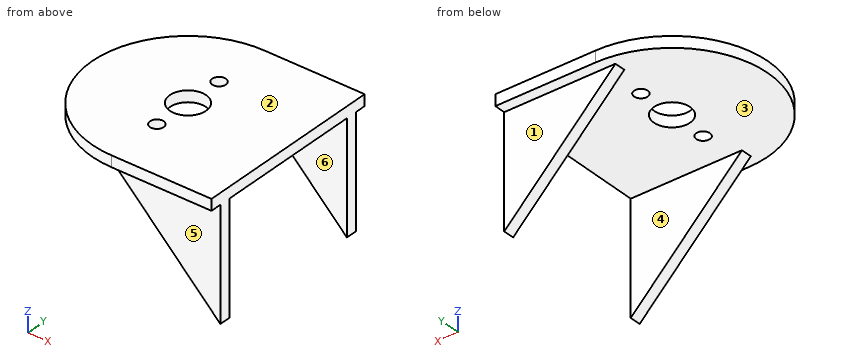
Autodesk Inventor part; units mm, degrees
ref_plane "YZ Plane" through (0, 0, 0) normal (1, 0, 0) x (0, 1, 0)
ref_plane "XZ Plane" through (0, 0, 0) normal (0, 1, 0) x (-1, 0, 0)
ref_plane "XY Plane" through (0, 0, 0) normal (0, 0, 1) x (1, 0, 0)
ref_plane "Płaszczyzna konstrukcyjna1" through (0, 0, 0) normal (0, 0, 1) x (1, 0, 0)
sketch "Szkic1" plane through (0, 0, 0) normal (0, 0, 1) x (1, 0, 0)
  circle A0 centre (0, 0) radius 12.25
  circle A1 centre (0, 7) radius 1.2295
  circle A2 centre (0, -7) radius 1.2295
  circle A3 centre (0, 0) radius 17.25
  line L0 (0, -17.25) -> (16, -17.25)
  line L1 (16, -17.25) -> (16, 17.25)
  line L2 (16, 17.25) -> (0, 17.25)
  line L3 (0, 17.25) -> (0, -17.25)
  point P0 (0, 0)
  dimension "d0" = 5
  dimension "d1" = 16
extrude "Wyciągnięcie proste1" add sketch "Szkic1" along normal blind 2
sketch "Szkic2" plane through (0, 0, 2) normal (0, 0, 1) x (1, 0, 0)
  arc A0 (-1.3229, 1.5) -> (1.3229, 1.5) centre (0, 0) ccw
  circle A1 centre (0, 7) radius 1.2295
  circle A2 centre (0, -7) radius 1.2295
  circle A3 centre (0, 0) radius 3.25
  point P0 (0, 0)
extrude "Wyciągnięcie proste2" cut sketch "Szkic2" against normal up to next
sketch "Szkic3" plane through (16, -17.25, 0) normal (1, 0, 0) x (0, 0, -1)
  line L0 (0, 0) -> (0, 10.8031)
  line L1 (0, 34.5) -> (-2, 34.5)
  line L2 (-2, 0) -> (-2, 10.8031)
  line L3 (0, 0) -> (-2, 0)
  line L4 (-2, 34.5) -> (-2, 34.5)
  line L5 (-2, 34.5) -> (-2, 0)
  line L6 (-2, 0) -> (-2, 0)
  line L7 (-2, 0) -> (-2, 34.5)
  line L8 (0, 0) -> (-2, 0)
  line L9 (-2, 34.5) -> (-2, 34.5)
  line L10 (-2, 34.5) -> (-2, 0)
  line L11 (-2, 0) -> (-2, 0)
  line L12 (-2, 0) -> (-2, 34.5)
  line L13 (0, 10.8031) -> (-2, 10.8031)
  line L14 (-2, 23.6969) -> (0, 23.6969)
  line L15 (0, 23.6969) -> (0, 34.5)
  line L16 (-2, 23.6969) -> (-2, 34.5)
  point P0 (0, 17.25)
  dimension "d6" = 0
  dimension "d9" = 0
extrude "Wyciągnięcie proste3" add sketch "Szkic3" along normal blind 2
sketch "Szkic5" plane through (0, 0, 2) normal (0, 0, 1) x (1, 0, 0)
  line L0 (0, 17.25) -> (18, 17.25)
  line L1 (0, -17.25) -> (18, -17.25)
  line L2 (0, -17.25) -> (18, -17.25)
  line L3 (18, 17.25) -> (9, 17.25)
  line L4 (9, 17.25) -> (9, -17.25)
  line L5 (9, -17.25) -> (18, -17.25)
  line L6 (18, -17.25) -> (18, 17.25)
  point P0 (0, 0)
extrude "Wyciągnięcie proste4" add sketch "Szkic5" against normal up to surface (2 mm away)
ref_plane "Płaszczyzna konstrukcyjna2" through (0, 14.25, 2) normal (0, 1, 0) x (1, 0, 0)
sketch "Szkic7" plane through (0, 14.25, 2) normal (0, 1, 0) x (1, 0, 0)
  line L0 (18, 2) -> (18, 22)
  line L1 (18, 2) -> (-2, 2)
  line L2 (-3.25, 2) -> (3.25, 2)
  line L3 (-2, 2) -> (18, 22)
  point P0 (0, 2)
  dimension "d28" = 20
  dimension "d29" = 20
extrude "Wyciągnięcie proste6" add sketch "Szkic7" along normal mid plane 2
mirror "Odbicie lustrzane1" about plane through (0, 0, 0) normal (0, 1, 0) of "Wyciągnięcie proste6"
ref_plane "Płaszczyzna konstrukcyjna3" through (0, 0, 0) normal (0, 1, 0) x (-1, 0, 0)
properties part number "console"
Input: part model. Units: mm. Frame: model coordinates. Face numbers are marked on the shaded views. A direction names the side the tool comes from. Give positions to 0.01 mm unless a question says otherwise; leave off trailing zeros. Order: outer loops, then holes, each group sorted by start corner. A loop starts at its lowest first (then second) coordinate and runs counter-clockwise, first axis right, second up. Notation, with made-up numbers: M 58,23.25 L 64,23.25 A38 cw 64,61.25 Z; hole C 9.25,69.25 d11. An arc over 180 degrees is marked long. One line per question, with ' | ' between items. Start each with the question number.
1. Section query D-D (x = 5.5). Return the cut outline in (y, z).
2. First-contact query: pin 1 Ø5 at (x, y) = (-2, -6) entering from -Z; pin 2 Ø5 at (x, y) = (0, 0) entering from +Z; pin 3 Ø10 at (x, z) = (7, -14) entering from +Y; pin 4 Ø10 at (x, z) = (10.5, -7.5) entering from -Y. Flat tips, straight axial feed; report the tip coordinate or a pass-through.
3. Pull-direction query (Y, two-part tool) for the marked faces 1, 2, 3 and 4; classes: released by +Y, released by -Y, zero draft, split by the parting line, or undercut.
4. Section query C-C (x = 13.5). Return the cut outline in (y, z).
5. Material intervals for probe 1 along Y at (x, z) = (0, 1); probe 2 along Y at (x, z) = (10.5, -9); probe 3 along Z at (x, y) = (13.5, 11), sorted ascending. Write a range as [from, to].
6. Section query A-A (y = 0). Return the cut outline in (x, z), and give its area (3 significant figures).
7. Access query for the marked faces 5 and 6. Directions: +Z, -Z, +X, -X, +Y, -Y. A direction counts if a zero-diameter tool reaches every point of the face in a straight line with its end or side. Return the directions, or none.
8. Section query B-B (z = -18.25). Return the cut outline in (x, y).
Here are the results:
1) outline: M -17.25,0 L -15.25,0 L -15.25,-7.5 L -13.25,-7.5 L -13.25,0 L 13.25,0 L 13.25,-7.5 L 15.25,-7.5 L 15.25,0 L 17.25,0 L 17.25,2 L -17.25,2 Z
2) pin 1: z = 0 | pin 2: through | pin 3: y = 15.25 | pin 4: y = -15.25
3) face 1: released by +Y | face 2: zero draft | face 3: undercut | face 4: undercut
4) outline: M -17.25,0 L -15.25,0 L -15.25,-15.5 L -13.25,-15.5 L -13.25,0 L 13.25,0 L 13.25,-15.5 L 15.25,-15.5 L 15.25,0 L 17.25,0 L 17.25,2 L -17.25,2 Z
5) probe 1: [-17.25, -8.23], [-5.77, -3.25], [3.25, 5.77], [8.23, 17.25] | probe 2: [-15.25, -13.25], [13.25, 15.25] | probe 3: [0, 2]
6) outline: M -17.25,0 L -3.25,0 L -3.25,2 L -17.25,2 Z; M 3.25,0 L 18,0 L 18,2 L 3.25,2 Z | area: 57.5 mm²
7) face 5: -Z, +X, -X, -Y | face 6: -Z, +X, -X
8) outline: M 16.25,-15.25 L 18,-15.25 L 18,-13.25 L 16.25,-13.25 Z; M 16.25,13.25 L 18,13.25 L 18,15.25 L 16.25,15.25 Z
